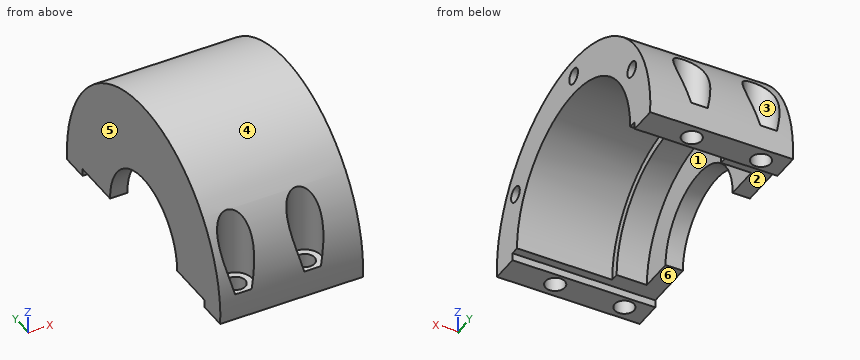
from build123d import *

# Parameters (mm, degrees)
F0_R           = 101.6
F1_DEPTH       = 104.775
F3_D           = 88.9
F3_CBORE_D     = 138.176
F3_CBORE_DEPTH = 92.075
F4_R           = 74.93
F5_DEPTH       = 69.85
F6_W           = 288.5075062513
F6_H           = 97.8503401275
F7_DEPTH       = 104.776
F8_W           = 80.9625
F8_H           = 28.0255991966
F9_DEPTH       = 104.776
F11_D          = 14.2875
F13_R          = 11.938
F14_DEPTH      = 88.1390001
F16_D          = 11.50874
F16_DEPTH      = 25.4
F16_TIP        = 3.4575743203


# Not quite as in the source:
# - a length typed as a fraction of an inch, garbled in the dataset ("3 / 203.2 mm" for 3/8 in), is restored


with BuildPart() as f1:
    # F0 (on Right) → F1 (new body)
    with BuildSketch(Plane.YZ):
        Circle(F0_R)
    extrude(amount=-F1_DEPTH)

    # F3 (through all)
    with Locations(Plane.YZ):
        with Locations((0, 0)):
            CounterBoreHole(F3_D / 2, F3_CBORE_D / 2, F3_CBORE_DEPTH)

    # F4 (on face) → F5 (cut)
    with BuildSketch(Plane.YZ):
        Circle(F4_R)
    extrude(amount=-F5_DEPTH, mode=Mode.SUBTRACT)

    # F6 (on face) → F7 (cut, through all)
    with BuildSketch(Plane.YZ):
        with Locations((9.2829242349, -54.5131700637)):
            Rectangle(F6_W, F6_H)
    extrude(amount=-F7_DEPTH, mode=Mode.SUBTRACT)

    # F8 (on face) → F9 (cut, through all)
    with BuildSketch(Plane.YZ):
        with Locations((-40.48125, -14.0127995983)):
            Rectangle(F8_W, F8_H)
        with Locations((40.48125, -14.0127995983)):
            Rectangle(F8_W, F8_H)
    extrude(amount=-F9_DEPTH, mode=Mode.SUBTRACT)

    # F11 (through all)
    with Locations(Plane(origin=(0, 0, -5.588), x_dir=(1, 0, 0), z_dir=(0, 0, -1))):
        with Locations((-36.576, 90.424), (-87.376, 90.424), (-36.576, -90.424), (-87.376, -90.424)):
            Hole(F11_D / 2)

    # F13 (on offset) → F14 (cut, through all)
    with BuildSketch(Plane(origin=(0, 0, 13.462), x_dir=(1, 0, 0), z_dir=(0, 0, -1))):
        with Locations((-87.376, 90.424)):
            Circle(F13_R)
        with Locations((-36.576, 90.424)):
            Circle(F13_R)
        with Locations((-87.376, -90.424)):
            Circle(F13_R)
        with Locations((-36.576, -90.424)):
            Circle(F13_R)
    extrude(amount=-F14_DEPTH, mode=Mode.SUBTRACT)

    # F16
    with Locations(Plane.YZ):
        with Locations((-76.9896583964, 44.45), (0, 88.9), (76.9896583964, 44.45)):
            Hole(F16_D / 2, depth=F16_DEPTH)
            with Locations((0, 0, -(F16_DEPTH + F16_TIP / 2))):  # 118° drill point
                Cone(0, F16_D / 2, F16_TIP, mode=Mode.SUBTRACT)


solid = f1.part
Can you work these out from the model? Positions are in its coordinate system, mm. Face numbers are marked on the shaded views. A direction names the side the tool comes from. Coordinates: 2 decimals unless noted, no trailing zeros. Loops run counter-clockwise (first coordinate to the right, second up) from the corner with the lowest first, then second, coordinate; pieces in that order, holes last. Notation, with made-up numbers: (76.25, 23.25) - (131.25, 23.25) arc R25 cw to (131.25, 62.25) - close; hole circle Ø7 at (32, -40). An arc over 180 degrees is marked (long way). Answer as a JSON object with one key per item and string values. Group by question number.
Item 1: If we section it at B-B (y = 46.5): List the corners of the cut face in (x, z) for me (3 decimals), plus the area to 3 significant figures.
Item 2: For pin 1 (18.5 mm diameter, centred on x = -87.376, y = -90.424, fed in from +Z); pin 2 (10 mm diameter, centred on x = -44, y = 28.5, fed in from +Z); pin 3 (1.5 mm diameter, centred on x = -31.5, z = 30.5, fed in from -Y), each with a flat end and sliding along its axis, tell me the tip position at first contact or that it passes through.
Item 3: On a 3-axis mill with a long thin cutter (end or side, diameter ignored), from which of +Z, -Z, +X, -X, +Y, -Y can I reach the whole of each face in a straight line? I mean the marked faces 1, 2 and 3. Say none if no direction works.
Item 4: If we mould it in two halves opening along Y, with no side actions, what happens to the marked faces 4, 5 and 6? For each: released by +Y, released by -Y, zero draft, split by the parting line, or undercut.
Item 5: If I drill on L1, parallel to Y at x = -99.5, z = 1; L2, parallel to Y at x = -77.5, z = 24; L3, parallel to Z at x = -26, y = 93, over which ranges is the centre line in solid material (lowest first)? Write a range as from..to.
Item 6: If we section it at D-D (x = -40.5): List the corners of the cut face in (y, z) for me.
Item 7: If we section it at A-A (x = -65): List the corners of the cut face in (y, z) for me.
Item 8: If we section it at C-C (z = 28.5): List the corners of the cut face in (x, y) for me (3 decimals).
Returned:
{
 "1": {"outline": "(-104.775, 0) - (-92.075, 0) - (-92.075, 51.097) - (-69.85, 51.097) - (-69.85, 58.756) - (0, 58.756) - (0, 90.334) - (-104.775, 90.334) - close", "area": "4,230 mm²"},
 "2": {"pin 1": "stops at z = 13.46", "pin 2": "stops at z = 98.84", "pin 3": "stops at y = -80"},
 "3": {"face 1": "-Z, +X", "face 2": "-Z, +X, -X", "face 3": "+Z"},
 "4": {"face 4": "split by the parting line", "face 5": "zero draft", "face 6": "undercut"},
 "5": {"L1": "y = -101.6..-44.44, 44.44..101.6", "L2": "y = -98.72..-97.13, -83.72..-64.79, 64.79..83.72, 97.13..98.72", "L3": "z = -5.59..13.46"},
 "6": {"outline": "(-101.45, -5.59) - (-96.39, -5.59) - (-96.39, 13.46) - (-100.7, 13.46) arc R101.6 ccw to start; (-84.45, -5.59) - (-80.96, -5.59) - (-80.96, 0) - (-74.93, 0) arc R74.93 cw to (74.93, 0) - (80.96, 0) - (80.96, -5.59) - (84.45, -5.59) - (84.45, 13.46) - (79.15, 13.46) - (79.15, 63.7) arc R101.6 ccw to (-79.15, 63.7) - (-79.15, 13.46) - (-84.45, 13.46) - close; (96.39, -5.59) - (101.45, -5.59) arc R101.6 ccw to (100.7, 13.46) - (96.39, 13.46) - close"},
 "7": {"outline": "(-101.45, -5.59) - (-80.96, -5.59) - (-80.96, 0) - (-74.93, 0) arc R74.93 cw to (74.93, 0) - (80.96, 0) - (80.96, -5.59) - (101.45, -5.59) arc R101.6 ccw (long way) to start"},
 "8": {"outline": "(-104.775, -97.521) - (-96.976, -97.521) arc R11.938 cw (long way) to (-77.776, -97.521) - (-46.176, -97.521) arc R11.938 cw (long way) to (-26.976, -97.521) - (0, -97.521) - (0, -69.298) - (-69.85, -69.298) - (-69.85, -62.936) - (-92.075, -62.936) - (-92.075, -34.111) - (-104.775, -34.111) - close; (-104.775, 34.111) - (-92.075, 34.111) - (-92.075, 62.936) - (-69.85, 62.936) - (-69.85, 69.298) - (0, 69.298) - (0, 97.521) - (-26.976, 97.521) arc R11.938 cw (long way) to (-46.176, 97.521) - (-77.776, 97.521) arc R11.938 cw (long way) to (-96.976, 97.521) - (-104.775, 97.521) - close"}
}
